Verification items for the finished model (mm, model axes). Give positions to 0.01 mm unless a question says otherwise; leave off trailing zeros. Answer as a JSON object with one key per item and string values. Group by question number.
(1) Thickness scan on line 1 (Y direction, x = 12, z = 35); line 2 (X direction, y = 26, z = 170.5); line 3 (Y direction, x = 6.5, z = 293). Record the ranges inside material, lowest first.
(2) Section check A-A (z = 187). Count the separate pieces of the cut face and the enclosed holes in it, then the cut area to 3 significant figures.
(3) Depth check by flat-ended pin: pin 1 Ø0.5 at (x, z) = (14, 187.5) entering from +Y; pin 2 Ø0.8 at (y, z) = (1, 243) entering from +X; pin 3 Ø0.5 at (y, z) = (29, 91) entering from -X. Enter the tip coordinate at first touch or a pass-through.
```python
from build123d import *

# Parameters (mm, degrees)
BOSCH_REXROTH_DIMENSION_30_8MM_SLOTS_3_DEPTH = 339


with BuildPart() as part:
    # Sketch1 → Bosch rexroth dimension 30 (8mm slots) 30X30(7) (new body)
    with BuildSketch(Plane(origin=(0, 15, 339), x_dir=(1, 0, 0), z_dir=(0, 0, -1))):
        with BuildLine():
            Line((6.00446543, 4.204465866), (6.00446543, -4.204465866))
            Line((6.00446543, -4.204465866), (10.049999564, -8.25))
            Line((10.049999564, -8.25), (12.59999928, -8.25))
            ThreePointArc((12.59999928, -8.25), (12.741420837, -8.191421273), (12.799999564, -8.049999716))
            Line((12.799999564, -8.049999716), (12.799999564, -4.649999613))
            ThreePointArc((12.799999564, -4.649999613), (12.975735606, -4.225735278), (13.39999994, -4.049999237))
            Line((13.39999994, -4.049999237), (15, -4.049999237))
            Line((15, -4.049999237), (15, -13.000000346))
            ThreePointArc((15, -13.000000346), (14.414213664, -14.414213664), (13.000000346, -15))
            Line((13.000000346, -15), (4.05, -15))
            Line((4.05, -15), (4.05, -13.399999434))
            ThreePointArc((4.05, -13.399999434), (4.225735989, -12.975735226), (4.650000197, -12.799999237))
            Line((4.650000197, -12.799999237), (8.049999924, -12.799999237))
            ThreePointArc((8.049999924, -12.799999237), (8.191421565, -12.741420475), (8.250000327, -12.599998834))
            Line((8.250000327, -12.599998834), (8.250000327, -10.049999237))
            Line((8.250000327, -10.049999237), (4.204466193, -6))
            Line((4.204466193, -6), (-4.204466193, -6))
            Line((-4.204466193, -6), (-8.250000327, -10.049999237))
            Line((-8.250000327, -10.049999237), (-8.250000327, -12.599998834))
            ThreePointArc((-8.250000327, -12.599998834), (-8.191421565, -12.741420475), (-8.049999924, -12.799999237))
            Line((-8.049999924, -12.799999237), (-4.650000197, -12.799999237))
            ThreePointArc((-4.650000197, -12.799999237), (-4.225735989, -12.975735226), (-4.05, -13.399999434))
            Line((-4.05, -13.399999434), (-4.05, -15))
            Line((-4.05, -15), (-13.000000346, -15))
            ThreePointArc((-13.000000346, -15), (-14.414213664, -14.414213664), (-15, -13.000000346))
            Line((-15, -13.000000346), (-15, -4.049999237))
            Line((-15, -4.049999237), (-13.39999994, -4.049999237))
            ThreePointArc((-13.39999994, -4.049999237), (-12.975735606, -4.225735278), (-12.799999564, -4.649999613))
            Line((-12.799999564, -4.649999613), (-12.799999564, -8.049999716))
            ThreePointArc((-12.799999564, -8.049999716), (-12.741420837, -8.191421273), (-12.59999928, -8.25))
            Line((-12.59999928, -8.25), (-10.049999564, -8.25))
            Line((-10.049999564, -8.25), (-6.00446543, -4.204465866))
            Line((-6.00446543, -4.204465866), (-6.00446543, 4.204465866))
            Line((-6.00446543, 4.204465866), (-10.049999564, 8.25))
            Line((-10.049999564, 8.25), (-12.59999928, 8.25))
            ThreePointArc((-12.59999928, 8.25), (-12.741420837, 8.191421273), (-12.799999564, 8.049999716))
            Line((-12.799999564, 8.049999716), (-12.799999564, 4.649999613))
            ThreePointArc((-12.799999564, 4.649999613), (-12.975735606, 4.225735278), (-13.39999994, 4.049999237))
            Line((-13.39999994, 4.049999237), (-15, 4.049999237))
            Line((-15, 4.049999237), (-15, 13.000000346))
            ThreePointArc((-15, 13.000000346), (-14.414213664, 14.414213664), (-13.000000346, 15))
            Line((-13.000000346, 15), (-4.05, 15))
            Line((-4.05, 15), (-4.05, 13.399999434))
            ThreePointArc((-4.05, 13.399999434), (-4.225735989, 12.975735226), (-4.650000197, 12.799999237))
            Line((-4.650000197, 12.799999237), (-8.049999924, 12.799999237))
            ThreePointArc((-8.049999924, 12.799999237), (-8.191421565, 12.741420475), (-8.250000327, 12.599998834))
            Line((-8.250000327, 12.599998834), (-8.250000327, 10.049999237))
            Line((-8.250000327, 10.049999237), (-4.204466193, 6))
            Line((-4.204466193, 6), (4.204466193, 6))
            Line((4.204466193, 6), (8.250000327, 10.049999237))
            Line((8.250000327, 10.049999237), (8.250000327, 12.599998834))
            ThreePointArc((8.250000327, 12.599998834), (8.191421565, 12.741420475), (8.049999924, 12.799999237))
            Line((8.049999924, 12.799999237), (4.650000197, 12.799999237))
            ThreePointArc((4.650000197, 12.799999237), (4.225735989, 12.975735226), (4.05, 13.399999434))
            Line((4.05, 13.399999434), (4.05, 15))
            Line((4.05, 15), (13.000000346, 15))
            ThreePointArc((13.000000346, 15), (14.414213664, 14.414213664), (15, 13.000000346))
            Line((15, 13.000000346), (15, 4.049999237))
            Line((15, 4.049999237), (13.39999994, 4.049999237))
            ThreePointArc((13.39999994, 4.049999237), (12.975735606, 4.225735278), (12.799999564, 4.649999613))
            Line((12.799999564, 4.649999613), (12.799999564, 8.049999716))
            ThreePointArc((12.799999564, 8.049999716), (12.741420837, 8.191421273), (12.59999928, 8.25))
            Line((12.59999928, 8.25), (10.049999564, 8.25))
            Line((10.049999564, 8.25), (6.00446543, 4.204465866))
        make_face()
        with BuildLine():
            Line((13.70000109, 12.700000408), (13.70000109, 10.499999626))
            ThreePointArc((13.70000109, 10.499999626), (13.407107874, 9.792892851), (12.7000011, 9.499999635))
            Line((12.7000011, 9.499999635), (10.500000318, 9.499999635))
            ThreePointArc((10.500000318, 9.499999635), (9.792893543, 9.792892851), (9.500000327, 10.499999626))
            Line((9.500000327, 10.499999626), (9.500000327, 12.700000408))
            ThreePointArc((9.500000327, 12.700000408), (9.792893543, 13.407107182), (10.500000318, 13.700000398))
            Line((10.500000318, 13.700000398), (12.7000011, 13.700000398))
            ThreePointArc((12.7000011, 13.700000398), (13.407107874, 13.407107182), (13.70000109, 12.700000408))
        make_face(mode=Mode.SUBTRACT)
        with BuildLine():
            Line((3.135929412, 4.518400903), (1.600129524, 3.280561767))
            ThreePointArc((1.600129524, 3.280561767), (0, 3.65), (-1.600129524, 3.280561767))
            Line((-1.600129524, 3.280561767), (-3.135929412, 4.518400903))
            ThreePointArc((-3.135929412, 4.518400903), (-3.881002259, 3.897155561), (-4.505336892, 3.154669473))
            Line((-4.505336892, 3.154669473), (-3.280561732, 1.600129597))
            ThreePointArc((-3.280561732, 1.600129597), (-3.65, 0), (-3.280561732, -1.600129597))
            Line((-3.280561732, -1.600129597), (-4.505336892, -3.154669473))
            ThreePointArc((-4.505336892, -3.154669473), (-3.881002259, -3.897155561), (-3.135929412, -4.518400903))
            Line((-3.135929412, -4.518400903), (-1.600129524, -3.280561767))
            ThreePointArc((-1.600129524, -3.280561767), (0, -3.65), (1.600129524, -3.280561767))
            Line((1.600129524, -3.280561767), (3.135929412, -4.518400903))
            ThreePointArc((3.135929412, -4.518400903), (3.881002259, -3.897155561), (4.505336892, -3.154669473))
            Line((4.505336892, -3.154669473), (3.280561732, -1.600129597))
            ThreePointArc((3.280561732, -1.600129597), (3.65, 0), (3.280561732, 1.600129597))
            Line((3.280561732, 1.600129597), (4.505336892, 3.154669473))
            ThreePointArc((4.505336892, 3.154669473), (3.881002259, 3.897155561), (3.135929412, 4.518400903))
        make_face(mode=Mode.SUBTRACT)
        with BuildLine():
            Line((-13.70000109, -12.700000408), (-13.70000109, -10.499999626))
            ThreePointArc((-13.70000109, -10.499999626), (-13.407107874, -9.792892851), (-12.7000011, -9.499999635))
            Line((-12.7000011, -9.499999635), (-10.500000318, -9.499999635))
            ThreePointArc((-10.500000318, -9.499999635), (-9.792893543, -9.792892851), (-9.500000327, -10.499999626))
            Line((-9.500000327, -10.499999626), (-9.500000327, -12.700000408))
            ThreePointArc((-9.500000327, -12.700000408), (-9.792893543, -13.407107182), (-10.500000318, -13.700000398))
            Line((-10.500000318, -13.700000398), (-12.7000011, -13.700000398))
            ThreePointArc((-12.7000011, -13.700000398), (-13.407107874, -13.407107182), (-13.70000109, -12.700000408))
        make_face(mode=Mode.SUBTRACT)
        with BuildLine():
            Line((10.500000318, -13.700000398), (12.7000011, -13.700000398))
            ThreePointArc((12.7000011, -13.700000398), (13.407107874, -13.407107182), (13.70000109, -12.700000408))
            Line((13.70000109, -12.700000408), (13.70000109, -10.499999626))
            ThreePointArc((13.70000109, -10.499999626), (13.407107874, -9.792892851), (12.7000011, -9.499999635))
            Line((12.7000011, -9.499999635), (10.500000318, -9.499999635))
            ThreePointArc((10.500000318, -9.499999635), (9.792893543, -9.792892851), (9.500000327, -10.499999626))
            Line((9.500000327, -10.499999626), (9.500000327, -12.700000408))
            ThreePointArc((9.500000327, -12.700000408), (9.792893543, -13.407107182), (10.500000318, -13.700000398))
        make_face(mode=Mode.SUBTRACT)
        with BuildLine():
            Line((-10.500000318, 13.700000398), (-12.7000011, 13.700000398))
            ThreePointArc((-12.7000011, 13.700000398), (-13.407107874, 13.407107182), (-13.70000109, 12.700000408))
            Line((-13.70000109, 12.700000408), (-13.70000109, 10.499999626))
            ThreePointArc((-13.70000109, 10.499999626), (-13.407107874, 9.792892851), (-12.7000011, 9.499999635))
            Line((-12.7000011, 9.499999635), (-10.500000318, 9.499999635))
            ThreePointArc((-10.500000318, 9.499999635), (-9.792893543, 9.792892851), (-9.500000327, 10.499999626))
            Line((-9.500000327, 10.499999626), (-9.500000327, 12.700000408))
            ThreePointArc((-9.500000327, 12.700000408), (-9.792893543, 13.407107182), (-10.500000318, 13.700000398))
        make_face(mode=Mode.SUBTRACT)
    extrude(amount=BOSCH_REXROTH_DIMENSION_30_8MM_SLOTS_3_DEPTH)


solid = part.part
```
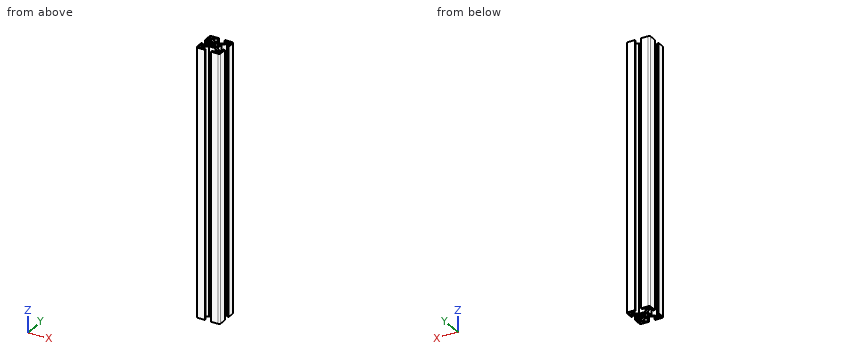
Solutions:
{
 "1": {"line 1": "y = 0 to 1.3, 5.5 to 6.75, 23.25 to 24.5, 28.7 to 30", "line 2": "x = -15 to -13.7, -9.5 to -8.25, 8.25 to 9.5, 13.7 to 15", "line 3": "y = 0 to 2.2, 6.7 to 10.3, 19.7 to 23.3, 27.8 to 30"},
 "2": {"separate pieces": "1", "enclosed holes": "5", "area": "317 mm2"},
 "3": {"pin 1": "stops at y = 29.85", "pin 2": "stops at x = 14.91", "pin 3": "stops at x = -14.85"}
}
